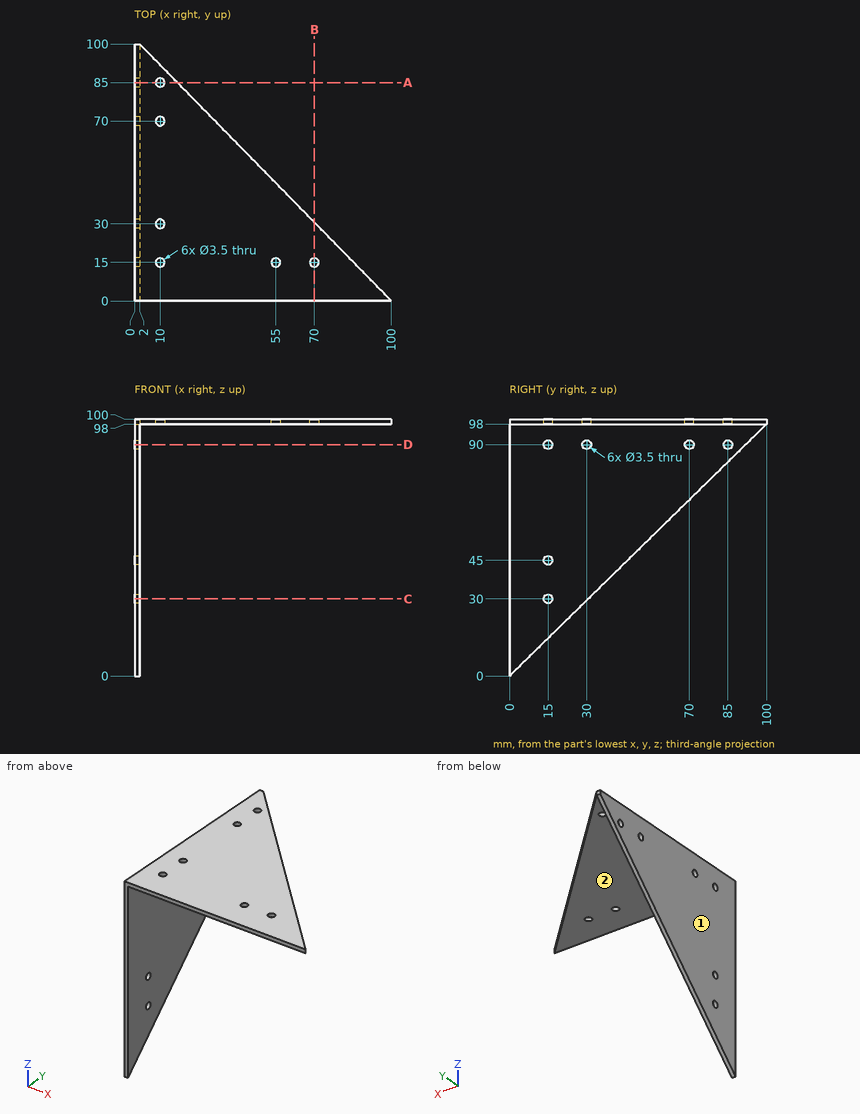
Here's the drawing with two shaded views (mm, measured from the low corner). I have some questions. A direction names the side the tool comes from. Coordinates: 2 decimals unless noted, no trailing zeros. Write each loop counter-clockwise with the first axis right and the second up, starting at its lowest first coordinate (ties: lowest second). Pieces come first, ordered by that corner, then holes.
Item 1: If I drill on line 1 (Z direction, x = 57, y = 30); line 2 (X direction, y = 62, z = 79.5); line 3 (Y direction, x = 55, z = 99.3), over which ranges is the centre line in solid material (lowest first)?
Item 2: I want a section at A-A on y = 85. Write out the boundary of the cut face in (x, z).
Item 3: On a 3-axis mill with a long thin cutter (end or side, diameter ignored), from which of +Z, -Z, +X, -X, +Y, -Y can I reach the whole of each face in a straight line? I mean the marked faces 1 and 2. Say none if no direction works.
Item 4: I want a section at C-C on z = 30. Write out the boundary of the cut face in (x, y), and give its area (3 significant figures).
Item 5: Will these pins go through, and if not, where does the flat tip stop? pin 1 (8 mm diameter, centred on x = 37.5, y = 26, fed in from -Z); pin 2 (5.5 mm diameter, centred on y = 15, z = 45, fed in from +X).
Item 6: I want a section at D-D on z = 90. Write out the boundary of the cut face in (x, y), and give its area (3 significant figures).
Item 7: I want a section at B-B on x = 70. Write out the boundary of the cut face in (y, z).
Findings below:
1. line 1: z = 98 to 100
1. line 2: x = 0 to 2
1. line 3: y = 0 to 13.25, 16.75 to 45.92
2. outline: (0, 83.3) - (2, 83.3) - (2, 88.25) - (0, 88.25) - close; (0, 91.75) - (2, 91.75) - (2, 98) - (8.25, 98) - (8.25, 100) - (0, 100) - close; (11.75, 98) - (16.7, 98) - (16.7, 100) - (11.75, 100) - close
3. face 1: +Z, -Z, -X, +Y, -Y
3. face 2: -Z, +X, +Y, -Y
4. outline: (0, 0) - (2, 0) - (2, 13.25) - (0, 13.25) - close; (0, 16.75) - (2, 16.75) - (2, 30.61) - (0, 30.61) - close
4. area: 54.2 mm2
5. pin 1: stops at z = 98
5. pin 2: stops at x = 2
6. outline: (0, 0) - (2, 0) - (2, 13.25) - (0, 13.25) - close; (0, 16.75) - (2, 16.75) - (2, 28.25) - (0, 28.25) - close; (0, 31.75) - (2, 31.75) - (2, 68.25) - (0, 68.25) - close; (0, 71.75) - (2, 71.75) - (2, 83.25) - (0, 83.25) - close; (0, 86.75) - (2, 86.75) - (2, 91.84) - (0, 91.84) - close
6. area: 156 mm2
7. outline: (0, 98) - (13.25, 98) - (13.25, 100) - (0, 100) - close; (16.75, 98) - (30.61, 98) - (30.61, 100) - (16.75, 100) - close
